The listing builds one solid part. Answer for the finished solid, in the listing's coordinates (mm). Face numbers are marked on the shaded views. A direction names the side the tool comes from. Give positions to 0.01 mm unless a question says otherwise; leave off trailing zeros. Loops run counter-clockwise (first coordinate to the right, second up) from the corner with the lowest first, then second, coordinate; pieces in that order, holes last. Notation, with made-up numbers: M 53.5,29.25 L 101.5,29.25 A14 cw 101.5,52.25 Z; hole C 37.5,7 d1. An arc over 180 degrees is marked long. Return JSON: item names as keys, results as strings.
from build123d import *

# Parameters (mm, degrees)
SKETCH1_R           = 2.5
BOSS_EXTRUDE1_DEPTH = 3
REVOLVE1_ANGLE      = 180
SKETCH3_R           = 2.5
BOSS_EXTRUDE2_DEPTH = 3


with BuildPart() as part:
    # Sketch1 → Boss-Extrude1 (new body)
    with BuildSketch(Plane(origin=(0, 0, 0), x_dir=(1, 0, 0), z_dir=(0, 1, 0))):
        Circle(SKETCH1_R)
    extrude(amount=BOSS_EXTRUDE1_DEPTH)

    # Sketch2 → Revolve1 (revolve)
    with BuildSketch(Plane(origin=(0, 3, 0), x_dir=(1, 0, 0), z_dir=(0, 1, 0))):
        with BuildLine():
            Line((0, -6), (0, 6))
            ThreePointArc((0, 6), (6, 0), (0, -6))
        make_face()
    revolve(axis=Axis((0, 3, 6), (0, 0, 1)), revolution_arc=REVOLVE1_ANGLE)

    # Sketch3 → Boss-Extrude2 (add)
    with BuildSketch(Plane.XZ):
        Circle(SKETCH3_R)
    extrude(amount=BOSS_EXTRUDE2_DEPTH)


solid = part.part
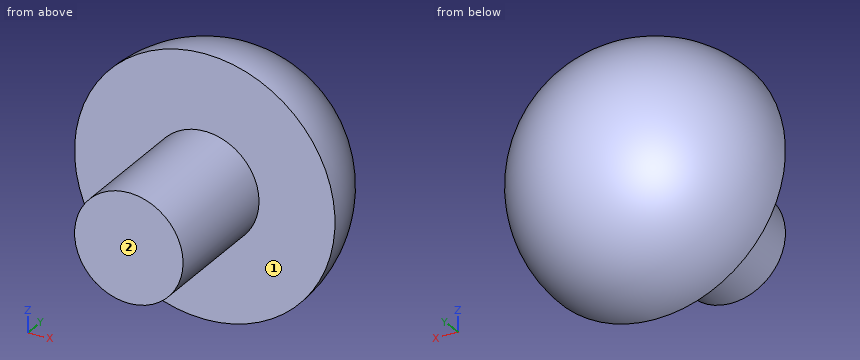
(1) The part is cut by section C-C (y = 0). Determine the outline of the cut face in (x, z).
Values follow:
{"outline": "C 0,0 d5"}
(2) The part is cut by section B-B (x = 0). Determine the outline of the cut face in (y, z).
Values follow:
{"outline": "M -3,-2.5 L 3,-2.5 L 3,-6 A6 ccw 3,6 L 3,2.5 L -3,2.5 Z"}
(3) The part is cut by section D-D (z = 3.5). Determine the outline of the cut face in (x, y).
Values follow:
{"outline": "M -4.87,3 L 4.87,3 A4.87 ccw Z"}
(4) A tool of negligible diameter and unlimited length cuts with its end or side. For the marked faces 1 and 2, from which of +Z, -Z, +X, -X, +Y, -Y can it reach the whole face along a straight path? Write none if from no direction.
Values follow:
{"face 1": "-Y", "face 2": "+Z, -Z, +X, -X, -Y"}
(5) Given pin 1 (4 mm diameter, centred on x = 3, y = 1.5, fed in from -Z); pin 2 (2 mm diameter, centred on y = 1.5, z = -4.5, fed in from -X); pin 3 (1.5 mm diameter, centred on x = 3, z = 4.5, fed in from -Y); pin 4 (3 mm diameter, centred on y = 0.5, z = -3.5, fed in from +X), each flat-ended and moving along its own axis, determine where each tip first touches the part or whether it passes through.
Values follow:
{"pin 1": "z = -5.76", "pin 2": "through", "pin 3": "y = 3", "pin 4": "x = 1.5"}
(6) The part is cut by section A-A (z = 0). Determine the outline of the cut face in (x, y), and give its area (3 significant figures).
Values follow:
{"outline": "M -6,3 L -2.5,3 L -2.5,-3 L 2.5,-3 L 2.5,3 L 6,3 A6 ccw Z", "area": "86.5 mm²"}
(7) Straight lines are drawn through the part: line 1 along Y through (x, z) = (-3.5, 0); line 2 along Z through (x, y) = (-2, 5.5); line 3 along Y through (x, z) = (1, 4.75). For each, find the intervals that lie inside material, in ascending order.
Values follow:
{"line 1": "3 to 7.87", "line 2": "-5.07 to 5.07", "line 3": "3 to 6.53"}
